Can you work these out from the model? Positions are in its coordinate system, mm. Face numbers are marked on the shaded views. A direction names the side the tool comes from. Give positions to 0.01 mm unless a question says otherwise; leave off trailing zeros. Order: outer loops, then holes, each group sorted by start corner. A loop starts at its lowest first (then second) coordinate and runs counter-clockwise, first axis right, second up. Notation, with made-up numbers: M -35,14 L -16,14 A19 ccw -16,33 Z; hole C 18.5,-35 d10. An arc over 180 degrees is marked long. One line per question, with ' | ' between items. Start each with the question number.
1) For the marked faces 5, 6, 7 and 8, which set-ups out of +Z, -Z, +X, -X, +Y, -Y let a thin tool reach every point of the face, with its end or its side?
2) If we section it at A-A, the plane y = 0: Please give me the cut outline in (x, z).
3) If we section it at C-C, the plane z = 6: Please give me the cut outline in (x, y), plus the area to 3 significant figures.
4) If we section it at B-B, the plane x = -5: Please give me the cut outline in (y, z).
5) If we section it at D-D, the plane z = 2.25: Please give me the cut outline in (x, y), plus the area to 3 significant figures.
6) I'm going to push flat-ended pins straight in: pin 1 Ø1 at (y, z) = (1, 9.5) entering from +X; pin 2 Ø1.6 at (y, z) = (-1, 5) entering from -X; pin 3 Ø0.8 at (y, z) = (-0.5, 6) entering from +X. Where does each tip first touch, or does it pass through?
7) Thinking about a two-plate mould opening in Y: for the marked faces 1, 2, 3 and 4, which applies, +Y half, -Y half, draft (parallel to the pull), parting line (faces both ways), or undercut?
8) Please list where these lines run through material, in increasing order: line 1 along Z through (x, y) = (-5.25, -2); line 2 along Y through (x, z) = (5.25, 10.25); line 3 along X through (y, z) = (2.3, 6). Write a range as [from, to].
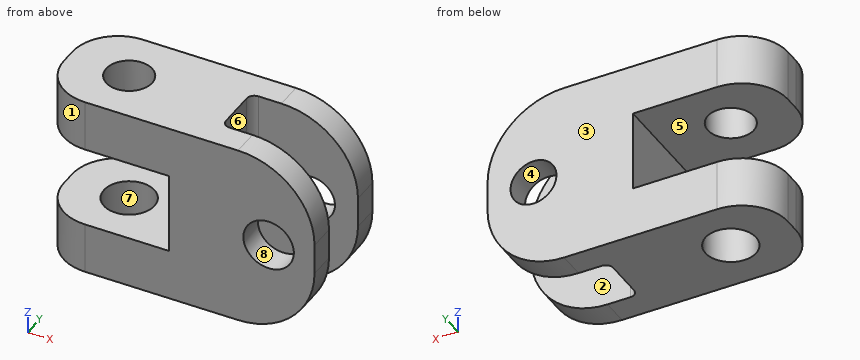
```python
from build123d import *

# Parameters (mm, degrees)
SKETCH_1_W          = 18
SKETCH_1_H          = 7
SKETCH_1_R          = 1.65
EXTRUDE_1_DEPTH     = 12
SKETCH_2_W          = 8.5
SKETCH_2_H          = 5.3
CUT_EXTRUDE_1_DEPTH = 12
SKETCH_3_W          = 14
SKETCH_3_H          = 3.5
CUT_EXTRUDE_2_DEPTH = 12
SKETCH_4_R          = 1.65
CUT_EXTRUDE_3_DEPTH = 12
FILLET_1_R          = 5
FILLET_2_R          = 3
FILLET_3_R          = 0.5
SKETCH_6_R          = 1.65
SKETCH_6_R_2        = 1.5
EXTRUDE_2_DEPTH     = 3.35
EXTRUDE_START       = -1.75
SKETCH_7_R          = 1.65
SKETCH_7_R_2        = 1.5
EXTRUDE_3_DEPTH     = 1.75


with BuildPart() as part:
    # 草图1 → 凸台-拉伸1 (new body)
    with BuildSketch(Plane.XY):
        Rectangle(SKETCH_1_W, SKETCH_1_H)
        with Locations((-5, 0)):
            Circle(SKETCH_1_R, mode=Mode.SUBTRACT)
    extrude(amount=EXTRUDE_1_DEPTH)

    # 草图2 → 切除-拉伸1 (cut)
    with BuildSketch(Plane(origin=(0, 3.5, 0), x_dir=(1, 0, 0), z_dir=(0, 1, 0))):
        with Locations((-4.75, -6)):
            Rectangle(SKETCH_2_W, SKETCH_2_H)
    extrude(amount=-CUT_EXTRUDE_1_DEPTH, mode=Mode.SUBTRACT)

    # 草图3 → 切除-拉伸2 (cut)
    with BuildSketch(Plane.XY.offset(12)):
        with Locations((9, 0)):
            Rectangle(SKETCH_3_W, SKETCH_3_H)
    extrude(amount=-CUT_EXTRUDE_2_DEPTH, mode=Mode.SUBTRACT)

    # 草图4 → 切除-拉伸3 (cut)
    with BuildSketch(Plane(origin=(0, 3.5, 0), x_dir=(1, 0, 0), z_dir=(0, 1, 0))):
        with Locations(Location((6, -6, 0), (0, 0, 270))):
            Circle(SKETCH_4_R)
    extrude(amount=-CUT_EXTRUDE_3_DEPTH, mode=Mode.SUBTRACT)

    # 圆角1
    fillet_1_edges = [part.edges().sort_by_distance(p)[0] for p in [
        (9, 2.625, 0),
        (9, 2.625, 12),
        (9, -2.625, 12),
        (9, -2.625, 0),
    ]]
    fillet(fillet_1_edges, radius=FILLET_1_R)

    # 圆角2
    fillet_2_edges = [part.edges().sort_by_distance(p)[0] for p in [
        (-9, -3.5, 1.675),
        (-9, 3.5, 1.675),
        (-9, -3.5, 10.325),
        (-9, 3.5, 10.325),
    ]]
    fillet(fillet_2_edges, radius=FILLET_2_R)

    # 圆角3
    fillet_3_edges = [part.edges().sort_by_distance(p)[0] for p in [
        (2, 1.75, 6),
        (2, -1.75, 6),
    ]]
    fillet(fillet_3_edges, radius=FILLET_3_R)

    # 草图6 → 凸台-拉伸2 (add)
    with BuildSketch(Plane(origin=(0, 0, 8.65), x_dir=(-1, 0, 0), z_dir=(0, 0, -1))):
        with Locations(Location((5, 0, 0), (0, 0, 180))):
            Circle(SKETCH_6_R)
        with Locations((5, 0)):
            Circle(SKETCH_6_R_2, mode=Mode.SUBTRACT)
    extrude(amount=-EXTRUDE_2_DEPTH)

    # 草图7 → 凸台-拉伸3 (add)
    with BuildSketch(Plane.XZ.offset(-1.75).offset(EXTRUDE_START)):
        with Locations(Location((6, 6, 0), (0, 0, 90))):
            Circle(SKETCH_7_R)
        with Locations(Location((6, 6, 0), (0, 0, 270))):
            Circle(SKETCH_7_R_2, mode=Mode.SUBTRACT)
    extrude(amount=EXTRUDE_3_DEPTH)


solid = part.part
```
Results found:
1) face 5: -X, +Y, -Y | face 6: +Z, -Z, +X | face 7: -Z | face 8: -Y
2) outline: M -9,0 L -6.65,0 L -6.65,3.35 L -9,3.35 Z; M -9,8.65 L -6.5,8.65 L -6.5,12 L -9,12 Z; M -3.5,8.65 L -0.5,8.65 L -0.5,3.35 L -3.35,3.35 L -3.35,0 L 2,0 L 2,12 L -3.5,12 Z
3) outline: M -0.5,-3.5 L 4.35,-3.5 L 4.35,-1.75 L 2.5,-1.75 A0.5 cw 2,-1.25 L 2,1.25 A0.5 cw 2.5,1.75 L 4.5,1.75 L 4.5,3.5 L -0.5,3.5 Z; M 7.5,1.75 L 9,1.75 L 9,3.5 L 7.5,3.5 Z; M 7.65,-3.5 L 9,-3.5 L 9,-1.75 L 7.65,-1.75 Z | area: 31.1 mm²
4) outline: M -3.5,0 L -1.65,0 L -1.65,3.35 L -3.5,3.35 Z; M -3.5,8.65 L -1.5,8.65 L -1.5,12 L -3.5,12 Z; M 1.5,8.65 L 3.5,8.65 L 3.5,12 L 1.5,12 Z; M 1.65,0 L 3.5,0 L 3.5,3.35 L 1.65,3.35 Z
5) outline: M -9,-0.5 A3 ccw -6,-3.5 L 8.18,-3.5 L 8.18,-1.75 L 2.5,-1.75 A0.5 cw 2,-1.25 L 2,1.25 A0.5 cw 2.5,1.75 L 8.18,1.75 L 8.18,3.5 L -6,3.5 A3 ccw -9,0.5 Z; hole C -5,0 d3.3 | area: 86.3 mm²
6) pin 1: stops at x = 2.07 | pin 2: stops at x = -0.5 | pin 3: stops at x = 2
7) face 1: -Y half | face 2: undercut | face 3: +Y half | face 4: draft
8) line 1: z = [0, 3.35], [8.65, 12] | line 2: y = [-3.5, -1.75], [1.75, 3.5] | line 3: x = [-0.5, 4.5], [7.5, 9]
